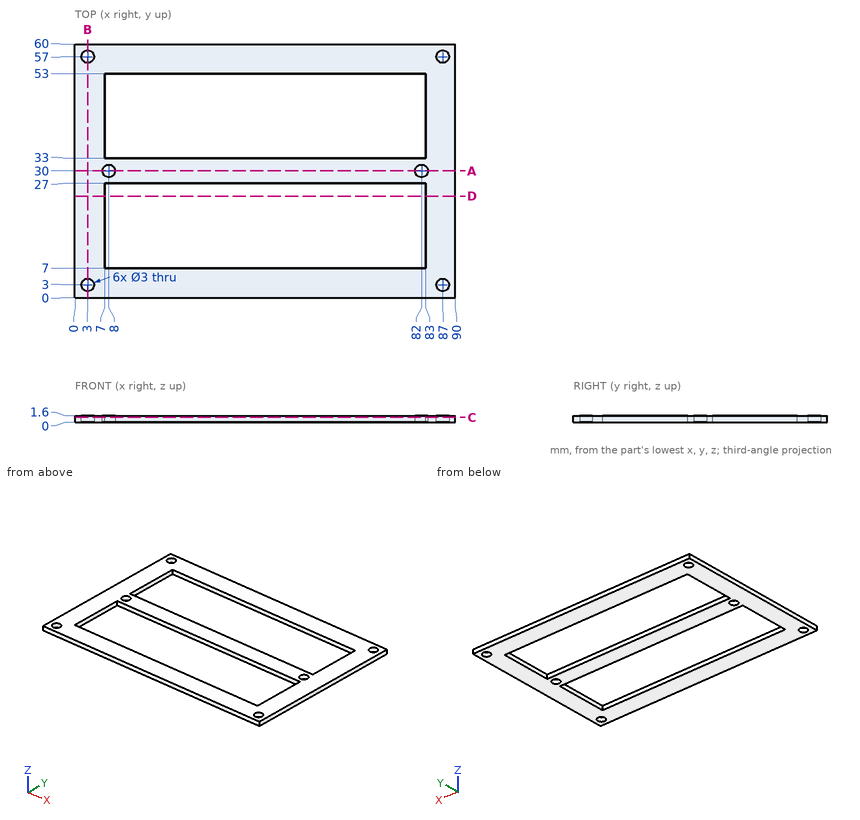
For this review, use the dimensioned drawing (mm, ordinates from the lowest corner) and the shaded views. Round coordinates to 2 decimals unless told otherwise and drop trailing zeros. Order: outer loops, then holes, each group sorted by start corner. A loop starts at its lowest first (then second) coordinate and runs counter-clockwise, first axis right, second up.
1) For L1, parallel to Y at x = 44, z = 0.5; L2, parallel to Y at x = 3, z = 0.6; L3, parallel to X at y = 22, z = 1.3, list the stretches that pass through material, from the lowest coordinate up.
The answers:
L1: y = 0 to 7, 27 to 33, 53 to 60
L2: y = 0 to 1.5, 4.5 to 55.5, 58.5 to 60
L3: x = 0 to 7, 83 to 90
2) Consider section A-A (y = 30). State the section outline as (x, z) points.
The answers:
outline: (0, 0) - (6.5, 0) - (6.5, 1.6) - (0, 1.6) - close; (9.5, 0) - (80.5, 0) - (80.5, 1.6) - (9.5, 1.6) - close; (83.5, 0) - (90, 0) - (90, 1.6) - (83.5, 1.6) - close
3) Consider section D-D (y = 24). State the section outline as (x, z) points, plus the area to 3 significant figures.
The answers:
outline: (0, 0) - (7, 0) - (7, 1.6) - (0, 1.6) - close; (83, 0) - (90, 0) - (90, 1.6) - (83, 1.6) - close
area: 22.4 mm2
4) Consider section B-B (x = 3). State the section outline as (y, z) points.
The answers:
outline: (0, 0) - (1.5, 0) - (1.5, 1.6) - (0, 1.6) - close; (4.5, 0) - (55.5, 0) - (55.5, 1.6) - (4.5, 1.6) - close; (58.5, 0) - (60, 0) - (60, 1.6) - (58.5, 1.6) - close
5) Consider section C-C (z = 1.2). Count the separate pieces of the cut face and the enclosed holes in it, plus the area to 3 significant figures.
The answers:
separate pieces: 1
enclosed holes: 8
area: 2,320 mm2
